from build123d import *

# Parameters (mm, degrees)
BOSS_EXTRUDE1_DEPTH     = 25
FILLET1_R               = 2
CUT_EXTRUDE1_DEPTH      = 171.565921027
CUT_EXTRUDE1_DEPTH_BACK = 171.565921027
SKETCH4_R               = 20
SKETCH4_R_2             = 16.5
SKETCH4_R_3             = 12.7
BOSS_EXTRUDE2_DEPTH     = 3


with BuildPart() as part:
    # Sketch1 → Revolve1 (revolve)
    with BuildSketch(Plane(origin=(0, 0, 0), x_dir=(0, 0, -1), z_dir=(1, 0, 0)), mode=Mode.PRIVATE) as revolve1_sk:
        Polygon((112.672204387, 118.557087119), (-15.352803504, 95.982824023), (-16.01266658, 99.725093484), (112.012341312, 122.299356581), align=None)
    revolve(revolve1_sk.sketch.rotate(Axis((0, 83.475765559, 13.147471648), (0, 0.17364817766692353, -0.9848077530122092)), 180), axis=Axis((0, 83.475765559, 13.147471648), (0, 0.17364817766692353, -0.9848077530122092)))


with BuildPart() as body_2:
    # Sketch2 → Boss-Extrude1 (new, symmetric)
    with BuildSketch(Plane(origin=(0, 0, 0), x_dir=(0, 0, -1), z_dir=(1, 0, 0))):
        Polygon((20.025829473, 108.41513389), (21.76231125, 98.56705636), (47.367312828, 103.081908979), (45.630831052, 112.929986509), align=None)
    extrude(amount=BOSS_EXTRUDE1_DEPTH, both=True)


with BuildPart() as body_3:
    # Mirror1: mirrored copy
    add(body_2.part.mirror(Plane(origin=(0, 83.207013304, 14.67164143), x_dir=(0, -0.17364817766692353, 0.9848077530122092), z_dir=(0, -0.9848077530122092, -0.17364817766692353))))


with BuildPart() as part_1:
    add(part.part)

    # Combine2: cut body 2, body 3
    add(body_2.part, mode=Mode.SUBTRACT)
    add(body_3.part, mode=Mode.SUBTRACT)

    # Fillet1
    fillet1_edges = [part_1.edges().sort_by_distance(p)[0] for p in [
        (-11.557199929, 98.56705636, -21.76231125),
        (11.557199929, 98.56705636, -21.76231125),
        (-11.557199929, 103.081908979, -47.367312828),
        (11.557199929, 103.081908979, -47.367312828),
        (-11.557199929, 81.234439907, -24.818519177),
        (11.557199929, 81.234439907, -24.818519177),
        (11.557199929, 85.749292526, -50.423520755),
        (-11.557199929, 85.749292526, -50.423520755),
    ]]
    fillet(fillet1_edges, radius=FILLET1_R)

    # Sketch3 → Cut-Extrude1 (cut, two sides)
    with BuildSketch(Plane(origin=(0, 0, 0), x_dir=(0, 0, -1), z_dir=(1, 0, 0))) as cut_extrude1_sk:
        with BuildLine():
            Line((-8.501269967, 85.919698853), (3.316423069, 88.003476985))
            ThreePointArc((3.316423069, 88.003476985), (5.169952558, 86.705621664), (3.872097237, 84.852092175))
            Line((3.872097237, 84.852092175), (-7.945595799, 82.768314043))
            ThreePointArc((-7.945595799, 82.768314043), (-9.799125288, 84.066169363), (-8.501269967, 85.919698853))
        make_face()
    extrude(amount=CUT_EXTRUDE1_DEPTH, mode=Mode.SUBTRACT)
    extrude(cut_extrude1_sk.sketch, amount=-CUT_EXTRUDE1_DEPTH_BACK, mode=Mode.SUBTRACT)

    # Sketch4 → Boss-Extrude2 (add)
    with BuildSketch(Plane(origin=(0, 0.268752256, -1.524169782), x_dir=(1, 0, 0), z_dir=(0, -0.17364817766692353, 0.9848077530122092))):
        with Locations(Location((0, 84.490615604, 0), (0, 0, 270))):
            Circle(SKETCH4_R)
        with Locations(Location((0, 84.490615604, 0), (0, 0, 270))):
            Circle(SKETCH4_R_2, mode=Mode.SUBTRACT)
        with Locations(Location((0, 84.490615604, 0), (0, 0, 270))):
            Circle(SKETCH4_R_2)
        with Locations(Location((0, 84.490615604, 0), (0, 0, 270))):
            Circle(SKETCH4_R_3, mode=Mode.SUBTRACT)
    extrude(amount=BOSS_EXTRUDE2_DEPTH)


solid = part_1.part
For this review, take the finished solid that the model builds, in its own axes (mm). A direction names the side the tool comes from. Give positions to 0.01 mm unless a question says otherwise; leave off trailing zeros. Order: outer loops, then holes, each group sorted by start corner. A loop starts at its lowest first (then second) coordinate and runs counter-clockwise, first axis right, second up. Notation, with made-up numbers: (62, -11) -> (66, -11) arc R22 ccw to (66, -1) -> close; hole circle Ø3 at (49, 16.25). An arc over 180 degrees is marked (long way). Write item = value, one per line.
1) For faces 1 (the face through (11.591, 83.465, -37.469)), 2 (the face through (14.91, 90.86, 14.45)), 3 (the face through (11.591, 100.798, -34.413)), 4 (the face through (0.175, 76.419, -25.668)), list the 3-axis set-ups (+Z, -Z, +X, -X, +Y, -Y) from which the entire face can be reached by the end or side of a thin tool; tool diameter is ignored.
Findings:
face_1 = +X, -X, -Y
face_2 = none
face_3 = +X, -X, +Y
face_4 = -Z, +X, -X
2) We need section A-A, the plane x = -1.5. Give the boundary of the cut face in (y, z), and give its area (3 significant figures).
Findings:
outline = (63.31, 12.64) -> (63.84, 9.68) -> (67.29, 10.29) -> (73.72, -26.14) -> (77.48, -25.48) -> (70.54, 13.91) -> close; (78.23, -51.75) -> (89.87, -117.73) -> (93.63, -117.07) -> (82, -51.09) -> close; (95.37, 18.29) -> (102.32, -21.1) -> (106.08, -20.44) -> (99.66, 16) -> (103.12, 16.61) -> (102.6, 19.57) -> close; (106.84, -46.71) -> (118.47, -112.69) -> (122.23, -112.02) -> (110.6, -46.04) -> close
area = 839 mm^2
3) To check wall thickness, follow L1, parallel to Y at x = 8.5, z = 11; L2, parallel to X at y = 78, z = 8; L3, parallel to X at y = 89, z = 8. State the ranges of each line that lie inside material, in increasing order. Write a range as from..to.
Findings:
L1 = 65.47..74.27, 93.44..98.21
L2 = -15.26..-11.03, 11.03..15.26
L3 = -15.86..-11.86, 11.86..15.86
4) We need section B-B, the plane x = 5. Give the boundary of the cut face in (y, z).
Findings:
outline = (63.88, 12.74) -> (64.41, 9.78) -> (67.99, 10.42) -> (74.42, -26.02) -> (78.4, -25.32) -> (71.46, 14.07) -> close; (78.93, -51.63) -> (90.56, -117.61) -> (94.55, -116.9) -> (82.92, -50.92) -> close; (94.45, 18.13) -> (101.4, -21.26) -> (105.39, -20.56) -> (98.96, 15.88) -> (102.55, 16.51) -> (102.03, 19.46) -> close; (105.91, -46.87) -> (117.55, -112.85) -> (121.54, -112.15) -> (109.9, -46.16) -> close
5) Draft analysis for pull direction X (two halves, no side actions). For faces 5 (the face through (14.638, 87.423, -53.083)), 6 (the face through (14.484, 86.947, 2.675)), 7 (the face through (3.815, 82.735, -52.408)), state which applies: pulls with the +X half, pulls with the -X half, needs draft (parallel to the pull), parting line crosses it, or undercut.
Findings:
face_5 = parting line crosses it
face_6 = needs draft
face_7 = undercut
6) Insertion check: pin 1 (10 mm diameter, centred on y = 76, z = -26, fed in from +X); pin 2 (6 mm diameter, centred on y = 89, z = -44, fed in from -X); pin 3 (3 mm diameter, centred on x = 3, y = 92.5, fed in from -Z). Each pin has a flat end and moves straight along its axis. Give the tip position at first contact, or say it passes through.
Findings:
pin_1 = 13.72
pin_2 = -16.43
pin_3 = -117.53
